```python
from build123d import *

# Parameters (mm, degrees)
BOSS_EXTRUDE1_DEPTH           = 17
CUT_EXTRUDE2_DEPTH            = 35
CUT_EXTRUDE3_DEPTH            = 30.5
CUT_EXTRUDE4_DEPTH            = 61
SKETCH6_R                     = 4
CUT_EXTRUDE5_DEPTH            = 61
CUT_EXTRUDE6_START            = -12.79
SKETCH7_W                     = 3.3
SKETCH7_H                     = 14.201279548
CUT_EXTRUDE6_DEPTH            = 12.79
SKETCH8_R                     = 1.25
CUT_EXTRUDE7_DEPTH            = 61
SKETCH9_R                     = 2.25
SKETCH9_R_2                   = 1.25
EXTRUDE_THIN1_DEPTH           = 1.75
EXTRUDE_THIN1_TAPER           = -30
EXTRUDE_THIN1_OTHER_WAY_DEPTH = 1.75
EXTRUDE_THIN1_OTHER_WAY_TAPER = -30
SKETCH10_R                    = 1.25
CUT_EXTRUDE9_DEPTH            = 43.000727623
FILLET1_SIZE                  = 10
FILLET1_SIZE_2                = 2


with BuildPart() as part:
    # Sketch1 → Boss-Extrude1 (new body)
    with BuildSketch(Plane.XY):
        Polygon((0, 0), (-11.797217655, 13.195289144), (-15.907217655, 9.520753176), (-24.431873803, 19.055654202), (-31.066793203, 13.123719901), (-22.542137055, 3.588818875), (-25.606127924, 0.849464945), (-14.904077823, -11.120869896), (-24.464229858, -20.947751043), (-24.464229858, -31.437751043), (-18.864229858, -31.437751043), (-18.864229858, -22.577751043), (0.565770142, -22.577751043), (0.565770142, -31.437751043), (6.165770142, -31.437751043), (6.165770142, -20.857751043), align=None)
    extrude(amount=BOSS_EXTRUDE1_DEPTH)

    # Sketch3 → Cut-Extrude2 (cut)
    with BuildSketch(Plane(origin=(-4.11, -3.674535968, 0), x_dir=(0, 0, -1), z_dir=(0.7454965618132088, 0.6665094720442348, 0))):
        with BuildLine():
            Line((-1.11054508, 20.98073524), (-2.78, 17.7))
            Line((-2.78, 17.7), (0.68, 17.7))
            Line((0.68, 17.7), (0.68, 32.569121824))
            Line((0.68, 32.569121824), (-17, 32.569121824))
            Line((-17, 32.569121824), (-17, 30.49))
            Line((-17, 30.49), (-5.15, 30.49))
            ThreePointArc((-5.15, 30.49), (-1.285745078, 26.518907223), (-1.11054508, 20.98073524))
        make_face()
    extrude(amount=-CUT_EXTRUDE2_DEPTH, mode=Mode.SUBTRACT)

    # Sketch4 → Cut-Extrude3 (cut, symmetric)
    with BuildSketch(Plane(origin=(-18.864229858, 0, 0), x_dir=(0, 0, -1), z_dir=(1, 0, 0))):
        with BuildLine():
            Line((-17, -26.307751043), (-17, -22.577751043))
            Line((-17, -22.577751043), (-18.338911285, -22.577751043))
            Line((-18.338911285, -22.577751043), (-18.338911285, -32.309712135))
            Line((-18.338911285, -32.309712135), (1.137649959, -32.309712135))
            Line((1.137649959, -32.309712135), (1.137649959, -22.577751043))
            Line((1.137649959, -22.577751043), (0, -22.577751043))
            Line((0, -22.577751043), (0, -29.657751043))
            Line((0, -29.657751043), (-3.9, -29.657751043))
            ThreePointArc((-3.9, -29.657751043), (-8.65, -31.031297694), (-13.4, -29.657751043))
            add(Edge.make_bspline(
                [(-13.4, -29.657751043), (-15.541480272, -28.298487281), (-17, -26.307751043)],
                knots=[0, 0, 0, 1, 1, 1], degree=2))
        make_face()
    extrude(amount=CUT_EXTRUDE3_DEPTH, both=True, mode=Mode.SUBTRACT)

    # Sketch5 → Cut-Extrude4 (cut)
    with BuildSketch(Plane.ZY.offset(-0.565770142)):
        with BuildLine():
            Line((3.9, -29.657751043), (0, -29.657751043))
            Line((0, -29.657751043), (0, -20.947751043))
            ThreePointArc((0, -20.947751043), (1.01950945, -25.719388602), (3.9, -29.657751043))
        make_face()
    extrude(amount=-CUT_EXTRUDE4_DEPTH, mode=Mode.SUBTRACT)

    # Sketch6 → Cut-Extrude5 (cut)
    with BuildSketch(Plane.ZY.offset(24.464229858)):
        with Locations(Location((8.5, -25.657751043, 0), (0, 0, 270))):
            Circle(SKETCH6_R)
    extrude(amount=-CUT_EXTRUDE5_DEPTH, mode=Mode.SUBTRACT)

    # Sketch7 → Cut-Extrude6 (cut)
    with BuildSketch(Plane(origin=(-20.321873803, 22.73019017, 0), x_dir=(0.7454965618132092, 0.6665094720442343, 0), z_dir=(-0.6665094720442343, 0.7454965618132092, 0)).offset(CUT_EXTRUDE6_START)):
        with Locations((-9.963103897, -7.399360226)):
            Rectangle(SKETCH7_W, SKETCH7_H)
    extrude(amount=CUT_EXTRUDE6_DEPTH, mode=Mode.SUBTRACT)

    # Sketch8 → Cut-Extrude7 (cut)
    with BuildSketch(Plane(origin=(-10.7449194, -9.606470269, 0), x_dir=(0, 0, 1), z_dir=(-0.7454965618132091, -0.6665094720442345, 0))):
        with Locations(Location((8.2, 26.49, 0), (0, 0, 270))):
            Circle(SKETCH8_R)
    extrude(amount=-CUT_EXTRUDE7_DEPTH, mode=Mode.SUBTRACT)

    # Sketch9 → Extrude-Thin1 (add)
    with BuildSketch(Plane(origin=(-7.4274597, -6.640503118, 0), x_dir=(0, 0, 1), z_dir=(-0.7454965618132092, -0.6665094720442343, 0))):
        with Locations((8.2, 26.49)):
            Circle(SKETCH9_R)
        with Locations((8.2, 26.49)):
            Circle(SKETCH9_R_2, mode=Mode.SUBTRACT)
    extrude(amount=EXTRUDE_THIN1_DEPTH, taper=EXTRUDE_THIN1_TAPER)

    # Sketch9 → Extrude-Thin1 other way (add)
    with BuildSketch(Plane(origin=(-7.4274597, -6.640503118, 0), x_dir=(0, 0, 1), z_dir=(-0.7454965618132092, -0.6665094720442343, 0))):
        with Locations((8.2, 26.49)):
            Circle(SKETCH9_R)
        with Locations((8.2, 26.49)):
            Circle(SKETCH9_R_2, mode=Mode.SUBTRACT)
    extrude(amount=-EXTRUDE_THIN1_OTHER_WAY_DEPTH, taper=EXTRUDE_THIN1_OTHER_WAY_TAPER)

    # Sketch10 → Cut-Extrude9 (cut, through all)
    with BuildSketch(Plane(origin=(-4.11, -3.674535968, 0), x_dir=(0, 0, -1), z_dir=(0.7454965618132088, 0.6665094720442348, 0))):
        with Locations(Location((-8.2, 26.49, 0), (0, 0, 270))):
            Circle(SKETCH10_R)
    extrude(amount=-CUT_EXTRUDE9_DEPTH, mode=Mode.SUBTRACT)

    # Fillet1
    # an asymmetric fillet: 10, 2 mm, written as the material it takes off along each edge
    with BuildSketch(Plane(origin=(-5.794459757, 35.718391003, 17), x_dir=(0.6665094720442343, -0.7454965618132092, 0), z_dir=(-0.7454965618132092, -0.6665094720442343, 0))) as fillet1_piece_1:
        with BuildLine():
            Bezier((FILLET1_SIZE, 0), (0, 0), (0, -FILLET1_SIZE_2), weights=[1, 0.707106781, 1])
            Line((0, -FILLET1_SIZE_2), (0, 0))
            Line((0, 0), (FILLET1_SIZE, 0))
        make_face()
    extrude(amount=58.9, mode=Mode.SUBTRACT)


solid = part.part
```
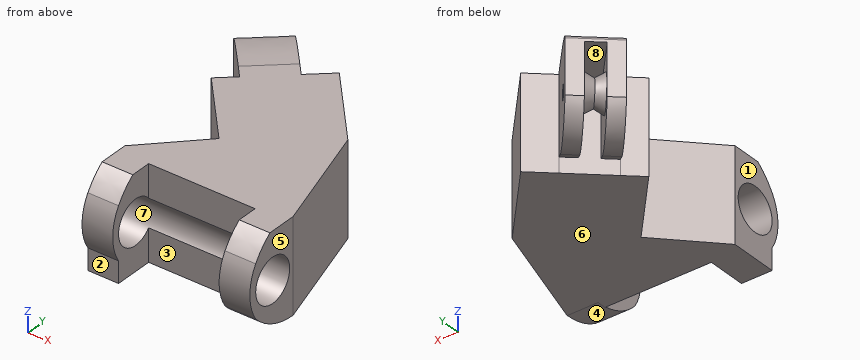
Geometry check sheet. Reference: the model listing, model coordinates, mm. Face numbers are marked on the shaded views. A direction names the side the tool comes from. Coordinates: 2 decimals unless noted, no trailing zeros. Loops run counter-clockwise (first coordinate to the right, second up) from the corner with the lowest first, then second, coordinate; pieces in that order, holes last. Notation, with made-up numbers: (-25.5, -34) -> (26.5, -34) arc R21 cw to (26.5, -19) -> close; hole circle Ø5 at (58.5, 40.25). An arc over 180 degrees is marked (long way). Put each result on its own line as item: value.
1) Release check for a two-part mould opening along Z. For the marked faces 5, 6, 7 and 8 record: released by +Z, released by -Z, zero draft, split by the parting line, or undercut.
Result set:
face 5: zero draft
face 6: released by -Z
face 7: undercut
face 8: undercut
2) Cross-section at A-A on y = 2.5. Record the boundary of the cut face in (x, z), plus the area to 3 significant figures.
Result set:
outline: (-23.76, 0) -> (-2.24, 0) -> (-2.24, 17) -> (-23.76, 17) -> close
area: 366 mm^2
3) Tool access check on the marked faces 1, 2, 3 and 4. Record the directions out of +Z, -Z, +X, -X, +Y, -Y that give a thin tool (end or side, any length) a straight path to the whole face; none if there is none.
Result set:
face 1: +Z, -Z, -X, -Y
face 2: -Z, +X, -X, -Y
face 3: +Z, -Z, -Y
face 4: -Z, +X, -Y
4) Gauge pin test, flat ends, axial feed: pin 1 Ø5.5 at (x, y) = (-25.5, 12) entering from -Z; pin 2 Ø3 at (y, z) = (-22.5, 6.5) entering from -X; pin 3 Ø3 at (x, z) = (-13.5, 2) entering from -Y. Record the tip position at first contact, or that the pin passes through.
Result set:
pin 1: stops at z = 0.68
pin 2: stops at x = -24.46
pin 3: stops at y = -22.58
5) Cross-section at B-B on y = -16.5. Record the boundary of the cut face in (x, z), plus the area to 3 significant figures.
Result set:
outline: (-20.14, 0) -> (4.88, 0) -> (4.88, 17) -> (-20.14, 17) -> close
area: 425 mm^2
6) Thickness scan on line 1 (Y direction, x = -21, z = 6.5); line 2 (Y direction, x = -16, z = 2); line 3 (Z direction, x = -6.5, y = -22). Record the ranges inside material, lowest first.
Result set:
line 1: y = -30.77 to -29.12, -22.19 to -17.39, -4.3 to 6.06, 11.02 to 15.22
line 2: y = -22.58 to -12.25, -9.9 to 9.44
line 3: z = 0 to 6.88, 10.12 to 17
